Input: part model. Units: mm. Frame: model coordinates. A direction names the side the tool comes from. Coordinates: 2 decimals unless noted, no trailing zeros. Order: outer loops, then holes, each group sorted by start corner. A loop starts at its lowest first (then second) coordinate and runs counter-clockwise, first axis right, second up.
from build123d import *

# Parameters (mm, degrees)
F1_DEPTH = 4
F2_DEPTH = 10
F3_W     = 8
F3_H     = 15
F4_DEPTH = 3


with BuildPart() as f1:
    # F0 (on Top) → F1 (new body)
    with BuildSketch(Plane.XY):
        with BuildLine():
            Line((23.5981723771, 50.6307036507), (29.1379201291, 63.6473221004))
            ThreePointArc((29.1379201291, 63.6473221004), (-69.3679635531, -9.3853946369), (45.0035054679, -53.6160842994))
            Line((45.0035054679, -53.6160842994), (35.576841855, -43.0654178585))
            ThreePointArc((35.576841855, -43.0654178585), (-55.4090369327, -7.0838208542), (23.5981723771, 50.6307036507))
        make_face()
        with BuildLine():
            Line((19.8677907274, 41.8655113026), (23.5981723771, 50.6307036507))
            ThreePointArc((23.5981723771, 50.6307036507), (-55.4090369327, -7.0838208542), (35.576841855, -43.0654178585))
            Line((35.576841855, -43.0654178585), (29.2286049616, -35.9602391123))
            ThreePointArc((29.2286049616, -35.9602391123), (-46.0089760191, -5.5339200114), (19.8677907274, 41.8655113026))
        make_face()
        with BuildLine():
            Line((14.5657325798, 29.407386674), (15.8289323737, 32.3754983065))
            ThreePointArc((15.8289323737, 32.3754983065), (-35.8310083049, -3.8557534328), (22.3545915501, -28.266592071))
            Line((22.3545915501, -28.266592071), (20.2043653008, -25.8599802663))
            ThreePointArc((20.2043653008, -25.8599802663), (-32.6475173449, -3.3308509117), (14.5657325798, 29.407386674))
        make_face()
        with BuildLine():
            Line((6.9658582886, 11.5501360659), (14.5657325798, 29.407386674))
            ThreePointArc((14.5657325798, 29.407386674), (-32.6475173449, -3.3308509117), (20.2043653008, -25.8599802663))
            Line((20.2043653008, -25.8599802663), (7.257370403, -11.3692303905))
            ThreePointArc((7.257370403, -11.3692303905), (-13.4870085006, -0.1715416686), (6.9658582886, 11.5501360659))
        make_face()
        with BuildLine():
            Line((15.8289323737, 32.3754983065), (19.8677907274, 41.8655113026))
            ThreePointArc((19.8677907274, 41.8655113026), (-46.0089760191, -5.5339200114), (29.2286049616, -35.9602391123))
            Line((29.2286049616, -35.9602391123), (22.3545915501, -28.266592071))
            ThreePointArc((22.3545915501, -28.266592071), (-35.8310083049, -3.8557534328), (15.8289323737, 32.3754983065))
        make_face()
        with BuildLine():
            ThreePointArc((32.4763517935, 45.4491855361), (28.1567060881, 48.2446037809), (23.5981723771, 50.6307036507))
            Line((23.5981723771, 50.6307036507), (19.8677907274, 41.8655113026))
            ThreePointArc((19.8677907274, 41.8655113026), (24.3303762174, 39.4396112828), (28.5006543682, 36.5398802079))
            Line((28.5006543682, 36.5398802079), (32.4763517935, 45.4491855361))
        make_face()
        with BuildLine():
            ThreePointArc((28.5006543682, 36.5398802079), (24.3303762174, 39.4396112828), (19.8677907274, 41.8655113026))
            Line((19.8677907274, 41.8655113026), (15.8289323737, 32.3754983065))
            ThreePointArc((15.8289323737, 32.3754983065), (20.1791178088, 29.8585196408), (24.1368343884, 26.7608149426))
            Line((24.1368343884, 26.7608149426), (28.5006543682, 36.5398802079))
        make_face()
        with BuildLine():
            ThreePointArc((35.6941134, 29.5530102292), (32.2869345127, 33.2416005149), (28.5006543682, 36.5398802079))
            Line((28.5006543682, 36.5398802079), (24.1368343884, 26.7608149426))
            ThreePointArc((24.1368343884, 26.7608149426), (25.022522536, 25.9345591175), (25.8799433339, 25.0790056366))
            Line((25.8799433339, 25.0790056366), (35.6941134, 29.5530102292))
        make_face()
        with BuildLine():
            ThreePointArc((44.6112733376, 33.6180930885), (38.9951173125, 39.9965338185), (32.4763517935, 45.4491855361))
            Line((32.4763517935, 45.4491855361), (28.5006543682, 36.5398802079))
            ThreePointArc((28.5006543682, 36.5398802079), (32.2869345127, 33.2416005149), (35.6941134, 29.5530102292))
            Line((35.6941134, 29.5530102292), (44.6112733376, 33.6180930885))
        make_face()
        with BuildLine():
            Line((22.3545915501, -28.266592071), (29.2286049616, -35.9602391123))
            ThreePointArc((29.2286049616, -35.9602391123), (32.8206282453, -32.7147750505), (36.0544716862, -29.1122863487))
            Line((36.0544716862, -29.1122863487), (29.0097989093, -21.3812899032))
            ThreePointArc((29.0097989093, -21.3812899032), (25.9119084265, -25.0459775688), (22.3545915501, -28.266592071))
        make_face()
        with BuildLine():
            Line((29.2286049616, -35.9602391123), (35.576841855, -43.0654178585))
            ThreePointArc((35.576841855, -43.0654178585), (39.2024865114, -39.7933027409), (42.5284655631, -36.2170057923))
            Line((42.5284655631, -36.2170057923), (36.0544716862, -29.1122863487))
            ThreePointArc((36.0544716862, -29.1122863487), (32.8206282453, -32.7147750505), (29.2286049616, -35.9602391123))
        make_face()
        with BuildLine():
            Line((36.0544716862, -29.1122863487), (42.5284655631, -36.2170057923))
            ThreePointArc((42.5284655631, -36.2170057923), (52.4212879012, -19.2963848035), (55.860020513, 0))
            ThreePointArc((55.860020513, 0), (54.3029220862, 13.0971197067), (49.7184350628, 25.4640748234))
            Line((49.7184350628, 25.4640748234), (41.1278773135, 21.3529354587))
            ThreePointArc((41.1278773135, 21.3529354587), (45.0185527566, 10.9899978491), (46.3405885269, 0))
            ThreePointArc((46.3405885269, 0), (43.6934524957, -15.4380165186), (36.0544716862, -29.1122863487))
        make_face()
        with BuildLine():
            Line((29.0097989093, -21.3812899032), (36.0544716862, -29.1122863487))
            ThreePointArc((36.0544716862, -29.1122863487), (43.6934524957, -15.4380165186), (46.3405885269, 0))
            ThreePointArc((46.3405885269, 0), (45.0185527566, 10.9899978491), (41.1278773135, 21.3529354587))
            Line((41.1278773135, 21.3529354587), (31.8282165391, 16.9024442795))
            ThreePointArc((31.8282165391, 16.9024442795), (34.9696231307, 8.7093885424), (36.0378688421, 0))
            ThreePointArc((36.0378688421, 0), (34.2357950026, -11.253369772), (29.0097989093, -21.3812899032))
        make_face()
    extrude(amount=-F1_DEPTH)

    # F0 (on Top) → F2 (join)
    with BuildSketch(Plane.XY):
        with BuildLine():
            Line((23.5981723771, 50.6307036507), (29.1379201291, 63.6473221004))
            ThreePointArc((29.1379201291, 63.6473221004), (-69.3679635531, -9.3853946369), (45.0035054679, -53.6160842994))
            Line((45.0035054679, -53.6160842994), (35.576841855, -43.0654178585))
            ThreePointArc((35.576841855, -43.0654178585), (-55.4090369327, -7.0838208542), (23.5981723771, 50.6307036507))
        make_face()
        with BuildLine():
            Line((19.8677907274, 41.8655113026), (23.5981723771, 50.6307036507))
            ThreePointArc((23.5981723771, 50.6307036507), (-55.4090369327, -7.0838208542), (35.576841855, -43.0654178585))
            Line((35.576841855, -43.0654178585), (29.2286049616, -35.9602391123))
            ThreePointArc((29.2286049616, -35.9602391123), (-46.0089760191, -5.5339200114), (19.8677907274, 41.8655113026))
        make_face()
        with BuildLine():
            Line((6.9658582886, 11.5501360659), (14.5657325798, 29.407386674))
            ThreePointArc((14.5657325798, 29.407386674), (-32.6475173449, -3.3308509117), (20.2043653008, -25.8599802663))
            Line((20.2043653008, -25.8599802663), (7.257370403, -11.3692303905))
            ThreePointArc((7.257370403, -11.3692303905), (-13.4870085006, -0.1715416686), (6.9658582886, 11.5501360659))
        make_face()
        with BuildLine():
            Line((14.5657325798, 29.407386674), (15.8289323737, 32.3754983065))
            ThreePointArc((15.8289323737, 32.3754983065), (-35.8310083049, -3.8557534328), (22.3545915501, -28.266592071))
            Line((22.3545915501, -28.266592071), (20.2043653008, -25.8599802663))
            ThreePointArc((20.2043653008, -25.8599802663), (-32.6475173449, -3.3308509117), (14.5657325798, 29.407386674))
        make_face()
    extrude(amount=F2_DEPTH)

    # F3 (on face) → F4 (cut)
    with BuildSketch(Plane.XY):
        Polygon((37.9851715346, 35.276671204), (33.8525412993, 39.626541011), (29.0030042003, 30.8811427968), align=None)
        with Locations((45.2681102753, -1.745258756)):
            Rectangle(F3_W, F3_H)
    extrude(amount=-F4_DEPTH, mode=Mode.SUBTRACT)


solid = f1.part
Item 1: Cut plane A-A on z = 3.25. Return loops of the section in (x, y), then the cut area to 3 significant figures.
Response values:
outline: (6.97, 11.55) - (15.83, 32.38) arc R36.04 ccw (long way) to (22.35, -28.27) - (7.26, -11.37) arc R13.49 cw (long way) to start; (19.87, 41.87) - (29.14, 63.65) arc R70 ccw (long way) to (45, -53.62) - (29.23, -35.96) arc R46.34 cw (long way) to start
area: 8,250 mm2
Item 2: Access query for faces 5 (the face through (-13.476, -0.573, 3.098)), 6 (the face through (49.268, -2, -1)). Directions: +Z, -Z, +X, -X, +Y, -Y. A direction counts if a zero-diameter tool reaches every point of the face in a straight line with its end or side. Return the directions, or none.
Response values:
face 5: +Z, -Z
face 6: +Z
Item 3: Cut plane B-B on x = 0. Return loops of the section in (y, z).
Response values:
outline: (-70, -4) - (-13.49, -4) - (-13.49, 10) - (-36.04, 10) - (-36.04, 0) - (-46.34, 0) - (-46.34, 10) - (-70, 10) - close; (13.49, -4) - (70, -4) - (70, 10) - (46.34, 10) - (46.34, 0) - (36.04, 0) - (36.04, 10) - (13.49, 10) - close
Item 4: Draft query along X for faces 1 (the face through (37.226, -44.912, 4.458)), 2 (the face through (-69.617, -7.308, 2.902)), 3 (the face through (-22, 1, -4)), 4 (the face through (35, 10, 0)). Return one class per face: pulls with the +X half, pulls with the -X half, needs draft (parallel to the pull), parting line crosses it, or undercut.
Response values:
face 1: pulls with the +X half
face 2: parting line crosses it
face 3: needs draft
face 4: undercut
Item 5: Cut plane C-C on x = -33. Return loops of the section in (y, z).
Response values:
outline: (-61.73, -4) - (61.73, -4) - (61.73, 10) - (32.53, 10) - (32.53, 0) - (14.48, 0) - (14.48, 10) - (-14.48, 10) - (-14.48, 0) - (-32.53, 0) - (-32.53, 10) - (-61.73, 10) - close
Item 6: Pin query (flat end, axial travel): pin 1 Ø5 at (y, z) = (-53, 5) entering from -X; pin 2 Ø1 at (y, z) = (17.5, 5.5) entering from +X; pin 3 Ø8 at (y, z) = (-53.5, -1.5) entering from -X. Return the tip coordinate at first contact, or that it passes through.
Response values:
pin 1: stops at x = -48.47
pin 2: stops at x = 9.71
pin 3: stops at x = -49.49
Item 7: Ray query, probe 1 along Y at (x, z) = (0, 7.5); probe 2 along X at (y, z) = (0, 4.75); probe 3 along Y at (x, z) = (0, -2). Return the intervals inside material, ascending.
Response values:
probe 1: y = -70 to -46.34, -36.04 to -13.49, 13.49 to 36.04, 46.34 to 70
probe 2: x = -70 to -46.34, -36.04 to -13.49
probe 3: y = -70 to -13.49, 13.49 to 70
Item 8: Cut plane D-D on y = 58. Return loops of the section in (x, z).
Response values:
outline: (-39.19, -4) - (26.73, -4) - (26.73, 10) - (-39.19, 10) - close
